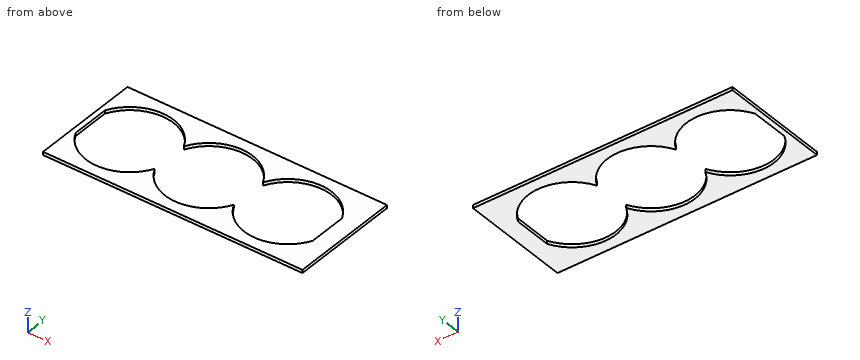
```python
from build123d import *

# Parameters (mm, degrees)
SKETCH4_W           = 330.2
SKETCH4_H           = 139.7
BOSS_EXTRUDE3_DEPTH = 4


with BuildPart() as part:
    # Sketch4 → Boss-Extrude3 (new body)
    with BuildSketch(Plane.XY):
        with Locations((165.1, 69.85)):
            Rectangle(SKETCH4_W, SKETCH4_H)
        with BuildLine():
            Line((6.35, 93.996304065), (6.35, 45.703695935))
            ThreePointArc((6.35, 45.703695935), (56.604, 14.096), (106.858, 45.703695935))
            Line((106.858, 45.703695935), (106.985, 45.703695935))
            ThreePointArc((106.985, 45.703695935), (157.239, 14.096), (207.493, 45.703695935))
            Line((207.493, 45.703695935), (207.62, 45.703695935))
            ThreePointArc((207.62, 45.703695935), (257.874, 14.096), (308.128, 45.703695935))
            Line((308.128, 45.703695935), (308.128, 93.996304065))
            ThreePointArc((308.128, 93.996304065), (257.874, 125.604), (207.62, 93.996304065))
            Line((207.62, 93.996304065), (207.493, 93.996304065))
            ThreePointArc((207.493, 93.996304065), (157.239, 125.604), (106.985, 93.996304065))
            Line((106.985, 93.996304065), (106.858, 93.996304065))
            ThreePointArc((106.858, 93.996304065), (56.604, 125.604), (6.35, 93.996304065))
        make_face(mode=Mode.SUBTRACT)
    extrude(amount=BOSS_EXTRUDE3_DEPTH)


solid = part.part
```
The listing builds one solid part. Answer for the finished solid, in the listing's coordinates (mm). Give positions to 0.01 mm unless a question says otherwise; leave off trailing zeros. Write each loop counter-clockwise with the first axis right and the second up, starting at its lowest first coordinate (ties: lowest second). Pieces come first, ordered by that corner, then holes. Notation, with made-up numbers: (25, 82) -> (59, 82) arc R22 cw to (59, 98) -> close; hole circle Ø5 at (-29.5, 66.5). An arc over 180 degrees is marked (long way). Write item = value, one per line. Start each with the question number.
1) The part is cut by section D-D, the plane y = 108.5. Determine the outline of the cut face in (x, z).
2) The part is cut by section C-C, the plane z = 3.4. Determine the outline of the cut face in (x, y) (3 decimals).
3) The part is cut by section B-B, the plane y = 49. Determine the outline of the cut face in (x, z).
4) The part is cut by section A-A, the plane x = 212. Determine the outline of the cut face in (y, z).
5) Straight lines are drawn through the part: line 1 along X through (y, z) = (67.5, 0.9); line 2 along X through (y, z) = (19.5, 1.7); line 3 along X through (y, z) = (20, 0.85). For each, find the intervals that lie inside material, in ascending order.
Solutions:
q1.outline = (0, 0) -> (16.42, 0) -> (16.42, 4) -> (0, 4) -> close; (96.79, 0) -> (117.06, 0) -> (117.06, 4) -> (96.79, 4) -> close; (197.42, 0) -> (217.69, 0) -> (217.69, 4) -> (197.42, 4) -> close; (298.06, 0) -> (330.2, 0) -> (330.2, 4) -> (298.06, 4) -> close
q2.outline = (0, 0) -> (330.2, 0) -> (330.2, 139.7) -> (0, 139.7) -> close; hole (6.35, 45.704) arc R55.754 ccw to (106.858, 45.704) -> (106.985, 45.704) arc R55.754 ccw to (207.493, 45.704) -> (207.62, 45.704) arc R55.754 ccw to (308.128, 45.704) -> (308.128, 93.996) arc R55.754 ccw to (207.62, 93.996) -> (207.493, 93.996) arc R55.754 ccw to (106.985, 93.996) -> (106.858, 93.996) arc R55.754 ccw to (6.35, 93.996) -> close
q3.outline = (0, 0) -> (6.35, 0) -> (6.35, 4) -> (0, 4) -> close; (308.13, 0) -> (330.2, 0) -> (330.2, 4) -> (308.13, 4) -> close
q4.outline = (0, 0) -> (38.16, 0) -> (38.16, 4) -> (0, 4) -> close; (101.54, 0) -> (139.7, 0) -> (139.7, 4) -> (101.54, 4) -> close
q5.line_1 = 0 to 6.35, 308.13 to 330.2
q5.line_2 = 0 to 32.66, 80.55 to 133.29, 181.18 to 233.93, 281.82 to 330.2
q5.line_3 = 0 to 31.63, 81.57 to 132.27, 182.21 to 232.9, 282.84 to 330.2
